from build123d import *

# Parameters (mm, degrees)
SKETCH1_W                      = 69.85
SKETCH1_H                      = 12.7
BOSS_EXTRUDE1_DEPTH            = 19.05
F_5_16_0_3125_DIAMETER_HOLE1_D = 7.9375
F_5_16_18_TAPPED_HOLE1_D       = 6.5278


with BuildPart() as part:
    # Sketch1 → Boss-Extrude1 (new body)
    with BuildSketch(Plane.XY):
        Rectangle(SKETCH1_W, SKETCH1_H)
    extrude(amount=BOSS_EXTRUDE1_DEPTH)

    # 5/16 (0.3125) Diameter Hole1 (through all)
    with Locations(Plane(origin=(0, 6.35, 0), x_dir=(1, 0, 0), z_dir=(0, 1, 0))):
        with Locations((-25.4, -9.525), (25.4, -9.525)):
            Hole(F_5_16_0_3125_DIAMETER_HOLE1_D / 2)

    # 5/16-18 Tapped Hole1 (through all)
    with Locations(Plane(origin=(0, 6.35, 0), x_dir=(1, 0, 0), z_dir=(0, 1, 0))):
        with Locations((0, -9.525)):
            Hole(F_5_16_18_TAPPED_HOLE1_D / 2)


solid = part.part
Geometry check sheet. Reference: the model listing, model coordinates, mm. Round coordinates to 2 decimals unless told otherwise and drop trailing zeros. Write each loop counter-clockwise with the first axis right and the second up, starting at its lowest first coordinate (ties: lowest second). Pieces come first, ordered by that corner, then holes. Notation, with made-up numbers: (-31.5, -22.5) - (-16.5, -22.5) arc R10 ccw to (-16.5, -7.5) - close; hole circle Ø5 at (15, 75). An arc over 180 degrees is marked (long way). One line per item, written item: value.
1. Mould release check, pull along X, two halves, no side actions. Record for faces 1 (the face through (-34.925, 0, 9)), 2 (the face through (-21.435, -0.089, 9.351)), 3 (the face through (0, -6.35, 14)), 4 (the face through (0.71, -0.09, 12.71)): released by +X, released by -X, zero draft, split by the parting line, or undercut.
The answers:
face 1: released by -X
face 2: undercut
face 3: zero draft
face 4: undercut
2. Scan lines: L1, parallel to X at y = 4.75, z = 9.5 (3 decimals); L2, parallel to Z at x = 0, y = -1; L3, parallel to X at y = 2.5, z = 8.75 (3 decimals). Record each from-to range of solid material in increasing order.
The answers:
L1: x = -34.925 to -29.369, -21.431 to -3.264, 3.264 to 21.431, 29.369 to 34.925
L2: z = 0 to 6.26, 12.79 to 19.05
L3: x = -34.925 to -29.292, -21.508 to -3.171, 3.171 to 21.508, 29.292 to 34.925
3. Cross-section at A-A on x = 0. Record the boundary of the cut face in (y, z), and give its area (3 significant figures).
The answers:
outline: (-6.35, 0) - (6.35, 0) - (6.35, 6.26) - (-6.35, 6.26) - close; (-6.35, 12.79) - (6.35, 12.79) - (6.35, 19.05) - (-6.35, 19.05) - close
area: 159 mm^2
4. Cross-section at B-B on y = -1. Give the number of separate pieces and of enclosed holes in the cut face, and give its area (3 significant figures).
The answers:
separate pieces: 1
enclosed holes: 3
area: 1,200 mm^2
5. Cross-section at C-C on z = 12. Record the boundary of the cut face in (x, y) (3 decimals).
The answers:
outline: (-34.925, -6.35) - (-28.502, -6.35) - (-28.502, 6.35) - (-34.925, 6.35) - close; (-22.298, -6.35) - (-2.128, -6.35) - (-2.128, 6.35) - (-22.298, 6.35) - close; (2.128, -6.35) - (22.298, -6.35) - (22.298, 6.35) - (2.128, 6.35) - close; (28.502, -6.35) - (34.925, -6.35) - (34.925, 6.35) - (28.502, 6.35) - close
6. Cross-section at D-D on x = 25.4. Record the boundary of the cut face in (y, z).
The answers:
outline: (-6.35, 0) - (6.35, 0) - (6.35, 5.56) - (-6.35, 5.56) - close; (-6.35, 13.49) - (6.35, 13.49) - (6.35, 19.05) - (-6.35, 19.05) - close
